```python
from build123d import *

# Parameters (mm, degrees)
F0_W      = 177.8
F0_H      = 228.6
F1_DEPTH  = 127
F2_W      = 38.1
F2_H      = 101.6
F3_DEPTH  = 177.8
F4_W      = 38.1
F4_H      = 101.6
F5_DEPTH  = 177.8
F6_R      = 6.199251325
F7_DEPTH  = 177.8
F8_W      = 165.1
F8_H      = 50.8
F9_DEPTH  = 101.6
F11_DEPTH = 174.498
F12_W     = 165.2032374404
F12_H     = 107.95
F13_DEPTH = 114.3
F15_R     = 5.6020191421
F16_DEPTH = 25.4
F17_R     = 5.6755182408
F18_DEPTH = 25.4
F19_R     = 6.2324496131
F20_DEPTH = 25.4
F21_R     = 6.232442208
F22_DEPTH = 25.4
F23_R     = 6.1943233013
F24_DEPTH = 25.4
F25_R     = 6.3267373896
F26_DEPTH = 25.4
F27_R     = 5.7686573469
F28_DEPTH = 25.4
F29_R     = 6.0099495699
F30_DEPTH = 25.4
F31_R     = 5.8905425669
F32_DEPTH = 25.4
F33_R     = 6.2038720929
F34_DEPTH = 25.4
F35_R     = 6.3267305002
F36_DEPTH = 25.4
F37_R     = 6.6105067138
F38_DEPTH = 25.4
F40_R     = 19.05
F40_R_2   = 10.1933204062
F41_DEPTH = 12.7
F42_W     = 177.6115447283
F42_H     = 126.4018714428
F43_DEPTH = 12.7


with BuildPart() as f1:
    # F0 (on Front) → F1 (new body)
    with BuildSketch(Plane.XZ):
        with Locations((88.9, 114.3)):
            Rectangle(F0_W, F0_H)
    extrude(amount=F1_DEPTH)

    # F2 (on face) → F3 (cut)
    with BuildSketch(Plane.YZ.offset(177.8)):
        with Locations((-107.95, 177.8)):
            Rectangle(F2_W, F2_H)
    extrude(amount=-F3_DEPTH, mode=Mode.SUBTRACT)

    # F4 (on face) → F5 (cut)
    with BuildSketch(Plane.YZ.offset(177.8)):
        with Locations((-19.05, 177.8)):
            Rectangle(F4_W, F4_H)
    extrude(amount=-F5_DEPTH, mode=Mode.SUBTRACT)

    # F6 (on face) → F7 (join)
    with BuildSketch(Plane(origin=(0, 0, 0), x_dir=(0, -1, 0), z_dir=(-1, 0, 0))):
        with Locations((61.0702037811, 211.2230211496)):
            Circle(F6_R)
    extrude(amount=-F7_DEPTH)

    # F8 (on face) → F9 (cut)
    with BuildSketch(Plane.XY.offset(228.6)):
        with Locations((88.9, -63.5)):
            Rectangle(F8_W, F8_H)
    extrude(amount=-F9_DEPTH, mode=Mode.SUBTRACT)

    # F10 (on face) → F11 (join)
    with BuildSketch(Plane.YZ.offset(177.8)):
        with BuildLine():
            Line((-63.5, 177.8), (-63.5, 187.9933204062))
            ThreePointArc((-63.5, 187.9933204062), (-70.707765982, 185.007765982), (-73.6933204062, 177.8))
            Line((-73.6933204062, 177.8), (-63.5, 177.8))
        make_face()
        with BuildLine():
            Line((-63.5, 167.6066795938), (-63.5, 177.8))
            Line((-63.5, 177.8), (-73.6933204062, 177.8))
            ThreePointArc((-73.6933204062, 177.8), (-70.707765982, 170.592234018), (-63.5, 167.6066795938))
        make_face()
        with BuildLine():
            Line((-53.3066795938, 177.8), (-63.5, 177.8))
            Line((-63.5, 177.8), (-63.5, 167.6066795938))
            ThreePointArc((-63.5, 167.6066795938), (-56.292234018, 170.592234018), (-53.3066795938, 177.8))
        make_face()
        with BuildLine():
            ThreePointArc((-53.3066795938, 177.8), (-56.292234018, 185.007765982), (-63.5, 187.9933204062))
            Line((-63.5, 187.9933204062), (-63.5, 177.8))
            Line((-63.5, 177.8), (-53.3066795938, 177.8))
        make_face()
    extrude(amount=-F11_DEPTH)

    # F12 (on face) → F13 (cut)
    with BuildSketch(Plane.XZ.offset(127)):
        with Locations((88.7493521441, 66.675)):
            Rectangle(F12_W, F12_H)
    extrude(amount=-F13_DEPTH, mode=Mode.SUBTRACT)

    # F15 (on face) → F16 (cut)
    with BuildSketch(Plane(origin=(0, 0, 0), x_dir=(1, 0, 0), z_dir=(0, 0, -1))):
        with Locations((83.3201929927, 88.2035493851)):
            Circle(F15_R)
    extrude(amount=-F16_DEPTH, mode=Mode.SUBTRACT)

    # F17 (on face) → F18 (cut)
    with BuildSketch(Plane(origin=(0, 0, 0), x_dir=(1, 0, 0), z_dir=(0, 0, -1))):
        with Locations((108.0974861979, 79.6003267169)):
            Circle(F17_R)
    extrude(amount=-F18_DEPTH, mode=Mode.SUBTRACT)

    # F19 (on face) → F20 (cut)
    with BuildSketch(Plane(origin=(0, 0, 0), x_dir=(1, 0, 0), z_dir=(0, 0, -1))):
        with Locations((91.0604074597, 70.961818099)):
            Circle(F19_R)
    extrude(amount=-F20_DEPTH, mode=Mode.SUBTRACT)

    # F21 (on face) → F22 (cut)
    with BuildSketch(Plane(origin=(0, 0, 0), x_dir=(1, 0, 0), z_dir=(0, 0, -1))):
        with Locations((69.7244107723, 74.4031071663)):
            Circle(F21_R)
    extrude(amount=-F22_DEPTH, mode=Mode.SUBTRACT)

    # F23 (on face) → F24 (cut)
    with BuildSketch(Plane(origin=(0, 0, 0), x_dir=(1, 0, 0), z_dir=(0, 0, -1))):
        with Locations((78.6717683077, 57.8849166632)):
            Circle(F23_R)
    extrude(amount=-F24_DEPTH, mode=Mode.SUBTRACT)

    # F25 (on face) → F26 (cut)
    with BuildSketch(Plane(origin=(0, 0, 0), x_dir=(1, 0, 0), z_dir=(0, 0, -1))):
        with Locations((108.9551225305, 62.0144642889)):
            Circle(F25_R)
    extrude(amount=-F26_DEPTH, mode=Mode.SUBTRACT)

    # F27 (on face) → F28 (cut)
    with BuildSketch(Plane(origin=(0, 0, 0), x_dir=(1, 0, 0), z_dir=(0, 0, -1))):
        with Locations((96.9106033444, 90.2330502868)):
            Circle(F27_R)
    extrude(amount=-F28_DEPTH, mode=Mode.SUBTRACT)

    # F29 (on face) → F30 (cut)
    with BuildSketch(Plane(origin=(0, 0, 0), x_dir=(1, 0, 0), z_dir=(0, 0, -1))):
        with Locations((93.8134491444, 55.1318824291)):
            Circle(F29_R)
    extrude(amount=-F30_DEPTH, mode=Mode.SUBTRACT)

    # F31 (on face) → F32 (cut)
    with BuildSketch(Plane(origin=(0, 0, 0), x_dir=(1, 0, 0), z_dir=(0, 0, -1))):
        with Locations((55.2709922194, 55.8201409876)):
            Circle(F31_R)
    extrude(amount=-F32_DEPTH, mode=Mode.SUBTRACT)

    # F33 (on face) → F34 (cut)
    with BuildSketch(Plane(origin=(0, 0, 0), x_dir=(1, 0, 0), z_dir=(0, 0, -1))):
        with Locations((72.4774450064, 41.3667224348)):
            Circle(F33_R)
    extrude(amount=-F34_DEPTH, mode=Mode.SUBTRACT)

    # F35 (on face) → F36 (cut)
    with BuildSketch(Plane(origin=(0, 0, 0), x_dir=(1, 0, 0), z_dir=(0, 0, -1))):
        with Locations((93.8134491444, 38.6136882007)):
            Circle(F35_R)
    extrude(amount=-F36_DEPTH, mode=Mode.SUBTRACT)

    # F37 (on face) → F38 (cut)
    with BuildSketch(Plane(origin=(0, 0, 0), x_dir=(1, 0, 0), z_dir=(0, 0, -1))):
        with Locations((113.7729287148, 46.8727871776)):
            Circle(F37_R)
    extrude(amount=-F38_DEPTH, mode=Mode.SUBTRACT)

    # F40 (on offset) → F41 (join, symmetric)
    with BuildSketch(Plane.YZ.offset(88.9)):
        with Locations((-63.5, 177.8)):
            Circle(F40_R)
        with Locations((-63.5, 177.8)):
            Circle(F40_R_2, mode=Mode.SUBTRACT)
    extrude(amount=F41_DEPTH, both=True)

    # F42 (on face) → F43 (join)
    with BuildSketch(Plane(origin=(0, 0, 0), x_dir=(1, 0, 0), z_dir=(0, 0, -1))):
        with Locations((88.8057723641, 63.2009357214)):
            Rectangle(F42_W, F42_H)
    extrude(amount=F43_DEPTH)

    # F45 (on offset) → F46 (revolve, cut)
    with BuildSketch(Plane.XZ.offset(63.5)):
        Polygon((88.8730700588, 187.96), (92.71, 196.85), (85.0630700588, 196.85), align=None)
    revolve(axis=Axis((88.71205585, -63.5, 177.8), (1, 0, 0)), mode=Mode.SUBTRACT)


solid = f1.part
```
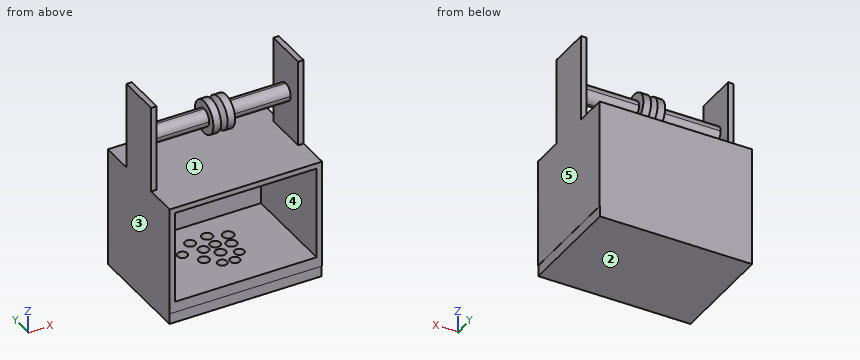
CAD build for the part. Positions are in the model's coordinates, mm. Face numbers are marked on the shaded views. A direction names the side the tool comes from. Coordinates: 2 decimals unless noted, no trailing zeros. Order: outer loops, then holes, each group sorted by start corner. A loop starts at its lowest first (then second) coordinate and runs counter-clockwise, first axis right, second up.
(1) Saw through at B-B, the plane y = -117.5. Write the cut outline in (x, z), and give its area (3 significant figures).
Solution:
outline: (0, -12.7) - (177.61, -12.7) - (177.61, 0) - (177.8, 0) - (177.8, 127) - (0, 127) - close; hole (6.15, 12.7) - (171.35, 12.7) - (171.35, 120.65) - (6.15, 120.65) - close
area: 7,000 mm2
(2) Drill centre lines: L1, parallel to Z at x = 146, y = -38; L2, parallel to Z at x = 139, y = -63.5; L3, parallel to X at y = -76, z = 212. Where is each one in solid material? Low to high.
Solution:
L1: z = -12.7 to 12.7, 120.65 to 127
L2: z = -12.7 to 12.7, 120.65 to 127, 167.61 to 187.99
L3: x = 0 to 6.35, 171.45 to 177.8
(3) Pin check, flat tips, straight feed: pin 1 Ø3.5 at (x, y) = (71.5, -40) entering from +Z; pin 2 Ø4 at (x, y) = (109.5, -62) entering from +Z; pin 3 Ø5 at (x, z) = (4, 166.5) entering from -Y. Stop position of each tip, or through.
Solution:
pin 1: stops at z = 127
pin 2: stops at z = 187.99
pin 3: stops at y = -88.9
(4) Saw through at A-A, the plane z = 156. Write the cut outline in (x, y), and give its area (3 significant figures).
Solution:
outline: (0, -88.9) - (6.35, -88.9) - (6.35, -38.1) - (0, -38.1) - close; (171.45, -88.9) - (177.8, -88.9) - (177.8, -38.1) - (171.45, -38.1) - close
area: 645 mm2
(5) Saw through at C-C, the plane x = 153. Write the cut outline in (y, z).
Solution:
outline: (-127, 0) - (-126.4, 0) - (-126.4, -12.7) - (0, -12.7) - (0, 127) - (-127, 127) - (-127, 120.65) - (-12.7, 120.65) - (-12.7, 12.7) - (-127, 12.7) - close; circle Ø20.39 at (-63.5, 177.8)
(6) Saw through at D-D, the plane y = -9. Write the cut outline in (x, z), and give its area (3 significant figures).
Solution:
outline: (0, -12.7) - (177.61, -12.7) - (177.61, 0) - (177.8, 0) - (177.8, 127) - (0, 127) - close
area: 24,800 mm2
(7) Mould opens along X. For the marked faces 1, 2 and 3 say: released by +X, released by -X, zero draft, split by the parting line, or undercut.
Solution:
face 1: undercut
face 2: zero draft
face 3: released by -X
(8) Which spindle directions (+Z, -Z, +X, -X, +Y, -Y) get a long thin tool onto all of the face, cutting with end or side? Do the marked faces 4 and 5. Say none if no direction does.
Solution:
face 4: -Y
face 5: +Z, -Z, +X, +Y, -Y
